The model under review builds one solid part; all positions refer to its coordinate system, in mm. Coordinates: 2 decimals unless noted, no trailing zeros. Order: outer loops, then holes, each group sorted by start corner. A loop starts at its lowest first (then second) coordinate and runs counter-clockwise, first axis right, second up.
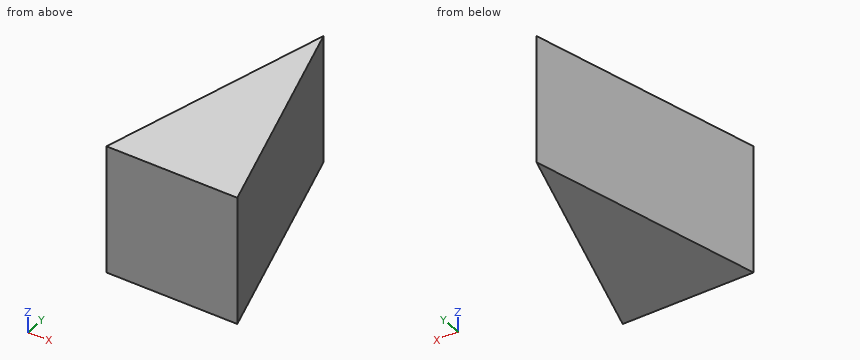
from build123d import *

# Parameters (mm, degrees)
F0_W      = 4
F0_H      = 7
F1_DEPTH  = 4
F6_DEPTH  = 25
F10_DEPTH = 25


with BuildPart() as f1:
    # F0 (on Top) → F1 (new body)
    with BuildSketch(Plane.XY):
        with Locations((2, 3.5)):
            Rectangle(F0_W, F0_H)
    extrude(amount=F1_DEPTH)

    # F5 (on 3pt) → F6 (cut)
    with BuildSketch(Plane(origin=(3.6981132075, 1.0566037736, 0), x_dir=(0.2747211279, -0.9615239476, 0), z_dir=(-0.9615239476, -0.2747211279, 0))):
        Polygon((9.2587498633, -3.3276440962), (7.0551056415, 9.7208032385), (-14.3242254853, 4.7958698124), (-11.358814391, -8.0770972366), align=None)
    extrude(amount=-F6_DEPTH, mode=Mode.SUBTRACT)

    # F9 (on 3pt) → F10 (cut)
    with BuildSketch(Plane(origin=(0, 0, 0), x_dir=(-0.2747211279, -0.9615239476, 0), z_dir=(-0.9615239476, 0.2747211279, 0))):
        Polygon((-10.4345437139, -9.9992519245), (-6.7709279247, -9.4136027619), (6.2972279266, -9.4136027619), (3.8799964823, 17.0888453722), (-6.9220042787, 14.663727954), (-10.4345437139, 17.9398357868), align=None)
    extrude(amount=F10_DEPTH, mode=Mode.SUBTRACT)


solid = f1.part
(1) Consider section A-A (z = 0.7). Give the boundary of the cut face in (x, y).
(2) Insertion check: pin 1 Ø2 at (x, z) = (1.5, 0.5) entering from +Y; pin 2 Ø1 at (y, z) = (5.5, 2) entering from -X. Each pin has a flat end and moves straight along its axis. Give the tip position at first contact, or say it passes through.
(3) Wall thickness on line 1 (X direction, y = 5.5, z = 0.6); line 2 (X direction, y = 2.25, z = 2.7): over which ranges is each line inside the solid? List them lowest first.
(4) Consider section B-B (x = 0.8). Give the boundary of the cut face in (y, z), then the cut area to 3 significant figures.
(5) Consider section C-C (y = 4.25). Give the boundary of the cut face in (x, z), then the cut area to 3 significant figures.
Findings:
1. outline: (0, 0) - (4, 0) - (2, 7) - close
2. pin 1: stops at y = 7
2. pin 2: stops at x = 1.43
3. line 1: x = 1.57 to 2.43
3. line 2: x = 0.64 to 3.36
4. outline: (0, 0) - (2.8, 0) - (2.8, 4) - (0, 4) - close
4. area: 11.2 mm2
5. outline: (1.21, 0) - (2.79, 0) - (2.79, 4) - (1.21, 4) - close
5. area: 6.29 mm2
